from build123d import *

# Parameters (mm, degrees)
F0_W      = 76.1575698853
F0_H      = 108.5386313498
F1_DEPTH  = 50.8
F3_DEPTH  = 118.872
F5_DEPTH  = 25.4
F6_R      = 12.5535289189
F7_DEPTH  = 5.08
F8_R      = 12.5680957502
F9_DEPTH  = 5.08
F10_R     = 13.425374539
F11_DEPTH = 12.7
F12_R     = 14.6312815901
F13_DEPTH = 12.7
F14_W     = 118.6601817608
F14_H     = 107.9017259181
F15_DEPTH = 50.8
F16_W     = 126.0260776617
F16_H     = 27.9104653746
F17_DEPTH = 12.7
F18_W     = 118.6601817608
F18_H     = 12.3918522149
F19_DEPTH = 143.764


with BuildPart() as f1:
    # F0 (on Top) → F1 (new body)
    with BuildSketch(Plane.XY):
        with Locations((38.0787849426, -12.8173213452)):
            Rectangle(F0_W, F0_H)
    extrude(amount=F1_DEPTH)

    # F2 (on face) → F3 (cut)
    with BuildSketch(Plane.XZ.offset(67.0866370201)):
        Polygon((76.1575698853, 50.8), (0, 50.8), (76.1575698853, 0), align=None)
    extrude(amount=-F3_DEPTH, mode=Mode.SUBTRACT)

    # F4 (on face) → F5 (cut)
    with BuildSketch(Plane.XZ.offset(67.0866370201)):
        Polygon((76.1575698853, 0), (24.0748073295, 34.7411864877), (24.0748073295, 0), align=None)
    extrude(amount=-F5_DEPTH, mode=Mode.SUBTRACT)

    # F6 (on face) → F7 (cut)
    with BuildSketch(Plane(origin=(23.4511739981, 0, 35.1571736743), x_dir=(0.8319076559, 0, -0.5549140943), z_dir=(0.5549140943, 0, 0.8319076559))):
        with Locations((42.292021215, -21.5434860438)):
            Circle(F6_R)
    extrude(amount=-F7_DEPTH, mode=Mode.SUBTRACT)

    # F8 (on face) → F9 (cut)
    with BuildSketch(Plane(origin=(23.4511739981, 0, 35.1571736743), x_dir=(0.8319076559, 0, -0.5549140943), z_dir=(0.5549140943, 0, 0.8319076559))):
        with Locations((41.7207404971, 16.4096038789)):
            Circle(F8_R)
    extrude(amount=-F9_DEPTH, mode=Mode.SUBTRACT)

    # F10 (on face) → F11 (cut)
    with BuildSketch(Plane(origin=(23.4511739981, 0, 35.1571736743), x_dir=(0.8319076559, 0, -0.5549140943), z_dir=(0.5549140943, 0, 0.8319076559))):
        with Locations((0, -21.8407977372)):
            Circle(F10_R)
    extrude(amount=-F11_DEPTH, mode=Mode.SUBTRACT)

    # F12 (on face) → F13 (cut)
    with BuildSketch(Plane(origin=(23.4511739981, 0, 35.1571736743), x_dir=(0.8319076559, 0, -0.5549140943), z_dir=(0.5549140943, 0, 0.8319076559))):
        with Locations((0, 17.1235315502)):
            Circle(F12_R)
    extrude(amount=-F13_DEPTH, mode=Mode.SUBTRACT)

    # F14 (on Top) → F15 (join)
    with BuildSketch(Plane.XY):
        with Locations((-59.3300908804, -13.0562540144)):
            Rectangle(F14_W, F14_H)
    extrude(amount=F15_DEPTH)

    # F16 (on face) → F17 (cut)
    with BuildSketch(Plane.XY.offset(50.8)):
        with Locations((-55.64714293, -13.9552326873)):
            Rectangle(F16_W, F16_H)
    extrude(amount=-F17_DEPTH, mode=Mode.SUBTRACT)

    # F18 (on face) → F19 (cut)
    with BuildSketch(Plane.XZ.offset(67.0071169734)):
        with Locations((-59.3300908804, 6.1959261075)):
            Rectangle(F18_W, F18_H)
    extrude(amount=-F19_DEPTH, mode=Mode.SUBTRACT)


solid = f1.part
Source: CAD feature listing. Evaluate the final solid. Frame: model axes, mm. A direction names the side the tool comes from. Give positions to 0.01 mm unless a question says otherwise; leave off trailing zeros. Write each loop counter-clockwise with the first axis right and the second up, starting at its lowest first coordinate (ties: lowest second). Pieces come first, ordered by that corner, then holes. Notation, with made-up numbers: (69.5, -18.75) - (99.5, -18.75) arc R19 ccw to (99.5, 3.25) - close; hole circle Ø4 at (-3.5, 68.5). An arc over 180 degrees is marked (long way). Write item = value, one per line. Start each with the question number.
Q1. Draft query along Z for faces 1 (the flat face through (-118.66, -14, 31)), 2 (the cylindrical face through (67.206, -17.773, 2.961)), 3 (the flat face through (-60, -14, 12.392)). Return one class per face: +Z half, -Z half, draft (parallel to the pull), parting line (faces both ways), or undercut.
Q2. Cut plane D-D, the plane y = -39.5. Return loops of the section in (x, z).
Q3. Cut plane C-C, the plane z = 24. Give the number of separate pieces and of enclosed holes in the cut face, then the cut area to 3 significant figures.
Q4. Cut plane B-B, the plane x = -52. Return loops of the section in (y, z).
Q5. Cut plane A-A, the plane y = -60. Return loops of the section in (x, z).
Q6. Reachability of faces 4 (the flat face through (-60, 40.895, 31)), 5 (the flat face through (38, -41.687, 10)), 6 (the flat face through (-60, -47, 50.8)), 7 (the flat face through (37.546, -1.517, 25.756)), 8 (the flat face through (16.23, 17.33, 24.71)) from +Z, -Z, +X, -X, +Y, -Y: full face, straight path, thin tool, end or side. Return the list, or none.
Q7. Material intervals for probe 1 along Y at (x, z) = (-65.5, 39.5); probe 2 along Z at (x, y) = (-25, -47.5); probe 3 along Y at (x, z) = (-22.5, 19), sorted ascending.
Q8. Pin query (flat end, axial travel): pin 1 Ø6.5 at (x, z) = (-48, 44.5) entering from -Y; pin 2 Ø6 at (y, z) = (-26, 37.5) entering from +X; pin 3 Ø19 at (x, z) = (-61.5, 22.5) entering from +Y; pin 4 Ø10 at (y, z) = (13.5, 11) entering from -X. Return the tip coordinate at first contact, or that it passes through.
Computed values:
q1.face_1 = draft
q1.face_2 = undercut
q1.face_3 = -Z half
q2.outline = (-118.66, 12.39) - (0, 12.39) - (0, 0) - (76.16, 0) - (0, 50.8) - (-118.66, 50.8) - close
q3.separate_pieces = 1
q3.enclosed_holes = 2
q3.area = 16,100 mm²
q4.outline = (-67.01, 12.39) - (40.89, 12.39) - (40.89, 50.8) - (0, 50.8) - (0, 38.1) - (-27.91, 38.1) - (-27.91, 50.8) - (-67.01, 50.8) - close
q5.outline = (-118.66, 12.39) - (0, 12.39) - (0, 0) - (24.07, 0) - (24.07, 34.74) - (0, 50.8) - (-118.66, 50.8) - close
q6.face_4 = +Z, -Z, -X, +Y
q6.face_5 = +Z, -Z, +X, -Y
q6.face_6 = +Z, +X, -X, +Y, -Y
q6.face_7 = +Z, +X, +Y, -Y
q6.face_8 = none
q7.probe_1 = -67.01 to -27.91, 0 to 40.89
q7.probe_2 = 12.39 to 50.8
q7.probe_3 = -67.01 to 40.89
q8.pin_1 = -67.01
q8.pin_2 = 12.17
q8.pin_3 = 40.89
q8.pin_4 = -118.66
